The listing builds one solid part. Answer for the finished solid, in the listing's coordinates (mm). Face numbers are marked on the shaded views. A direction names the side the tool comes from. Coordinates: 2 decimals unless noted, no trailing zeros. Write each loop counter-clockwise with the first axis right and the second up, starting at its lowest first coordinate (ties: lowest second). Pieces come first, ordered by that corner, then holes. Notation, with made-up numbers: M -23,37 L 5,37 A9 ccw 5,53 Z; hole C 22.25,-36.75 d11. An arc over 180 degrees is marked long. Answer as a JSON object with one key per item and string values. Group by question number.
from build123d import *

# Parameters (mm, degrees)
F1_DEPTH = 60
F2_W     = 70
F2_H     = 15
F3_DEPTH = 50
F4_R     = 15
F5_R     = 15
F6_DEPTH = 67.5
F7_SIZE  = 5
F8_SIZE  = 4.99999
F9_SIZE  = 5


# Not quite as in the source:
# - a fillet or chamfer is up to 0.001 mm smaller than in the source, because OpenCascade refuses the exact size


with BuildPart() as f1:
    # F0 (on Front) → F1 (new body)
    with BuildSketch(Plane.XZ):
        Polygon((-8.0390890029, 59.2476050396), (-48.0390890029, 59.2476050396), (-48.0390890029, -60.7523949604), (-8.0390890029, -60.7523949604), (-8.0390890029, -20.7523949604), (11.9609109971, -20.7523949604), (11.9609109971, -60.7523949604), (51.9609109971, -60.7523949604), (51.9609109971, 59.2476050396), (11.9609109971, 59.2476050396), (11.9609109971, 19.2476050396), (-8.0390890029, 19.2476050396), align=None)
    extrude(amount=F1_DEPTH)

    # F2 (on face) → F3 (cut)
    with BuildSketch(Plane.XZ.offset(60)):
        with Locations((1.9609109971, -0.7523949604)):
            Rectangle(F2_W, F2_H)
    extrude(amount=-F3_DEPTH, mode=Mode.SUBTRACT)

    # F4 (on face) + F5 (on face) → F6 (cut)
    with BuildSketch(Plane(origin=(0, 0, -60.7523949604), x_dir=(1, 0, 0), z_dir=(0, 0, -1))):
        with Locations((-28.0390890029, 20)):
            Circle(F4_R)
    with BuildSketch(Plane(origin=(0, 0, -60.7523949604), x_dir=(1, 0, 0), z_dir=(0, 0, -1))):
        with Locations((31.9609109971, 20)):
            Circle(F5_R)
    extrude(amount=-F6_DEPTH, mode=Mode.SUBTRACT)

    # F7
    f7_edges = [f1.edges().sort_by_distance(p)[0] for p in [
        (-48.039089, -30, 59.247605),
        (-8.039089, -30, 59.247605),
        (11.960911, -30, 59.247605),
        (51.960911, -30, 59.247605),
        (31.960911, -60, 59.247605),
        (-28.039089, -60, 59.247605),
        (31.960911, 0, 59.247605),
        (-28.039089, 0, 59.247605),
        (1.960911, -60, 6.747605),
        (-33.039089, -60, -0.752395),
        (1.960911, -60, -8.252395),
        (36.960911, -60, -0.752395),
        (51.960911, -60, -0.752395),
        (51.960911, 0, -0.752395),
        (11.960911, -60, 39.247605),
        (1.960911, -60, 19.247605),
        (-8.039089, -60, 39.247605),
        (31.960911, -60, -60.752395),
        (11.960911, -60, -40.752395),
        (-48.039089, -60, -0.752395),
        (1.960911, -60, -20.752395),
        (-28.039089, -60, -60.752395),
        (-8.039089, -60, -40.752395),
        (-48.039089, 0, -0.752395),
        (11.960911, 0, -40.752395),
        (-8.039089, 0, -40.752395),
        (11.960911, 0, 39.247605),
        (-8.039089, 0, 39.247605),
    ]]
    chamfer(f7_edges, length=F7_SIZE)

    # F8 (size 5 in the source; OpenCascade refuses exactly that, so slightly less here)
    f8_edges = [f1.edges().sort_by_distance(p)[0] for p in [
        (1.960911, 0, -20.752395),
    ]]
    chamfer(f8_edges, length=F8_SIZE)

    # F9
    f9_edges = [f1.edges().sort_by_distance(p)[0] for p in [
        (1.960911, 0, 19.247605),
    ]]
    chamfer(f9_edges, length=F9_SIZE)


solid = f1.part
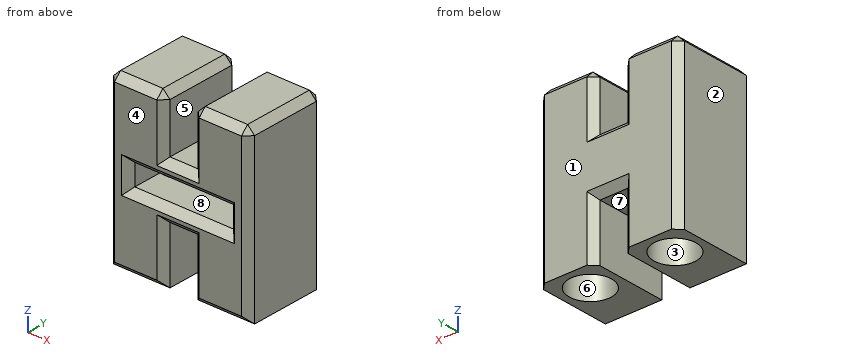
Item 1: Consider L1, parallel to X at y = -20, z = -32; L2, parallel to X at y = -20, z = -10.5; L3, parallel to X at y = -20, z = 19.5. Determine where each line is inside the solid, lowest interval first. Write a range as from..to.
Item 2: For a pull along Y with two mould halves and no side action, classify the marked faces 1, 2, 3 and 4 as +Y half, -Y half, draft (parallel to the pull), parting line (faces both ways), or undercut.
Item 3: A cutting plane is placed at C-C, the plane z = 30. Write down the section's boundary in (x, y), and give its area (3 significant figures).
Item 4: A cutting plane is placed at A-A, the plane z = -38. Write down the section's boundary in (x, y).
Item 5: A cutting plane is placed at B-B, the plane y = -20. Write down the section's boundary in (x, z).
Item 6: Flat-ended cylindrical pins translate along their axes: pin 1 Ø22 at (x, y) = (3, -40) entering from +Z; pin 2 Ø10 at (x, y) = (-3, -33.5) entering from -Z; pin 3 Ø12 at (x, z) = (-6.5, -3) entering from -Y. Find the tip coordinate at first contact, or state that the pin passes through.
Item 7: A tool of negligible diameter and unlimited length cuts with its end or side. For the marked faces 5, 6, 7 and 8, from which of +Z, -Z, +X, -X, +Y, -Y can it reach the whole face along a straight path? Write none if from no direction.
Item 8: A cutting plane is placed at D-D, the plane x = -29.5. Write down the section's boundary in (y, z).
Answer:
{
 "1": {"L1": "-48.04..-43.04, -13.04..-8.04, 11.96..16.96, 46.96..51.96", "L2": "-48.04..-43.04, -13.04..16.96, 46.96..51.96", "L3": "-48.04..-8.04, 11.96..51.96"},
 "2": {"face 1": "+Y half", "face 2": "draft", "face 3": "undercut", "face 4": "-Y half"},
 "3": {"outline": "M -48.04,-55 L -43.04,-60 L -13.04,-60 L -8.04,-55 L -8.04,-5 L -13.04,0 L -43.04,0 L -48.04,-5 Z; M 11.96,-55 L 16.96,-60 L 46.96,-60 L 51.96,-55 L 51.96,-5 L 46.96,0 L 16.96,0 L 11.96,-5 Z", "area": "4,700 mm2"},
 "4": {"outline": "M -48.04,-55 L -43.04,-60 L -13.04,-60 L -8.04,-55 L -8.04,-5 L -13.04,0 L -43.04,0 L -48.04,-5 Z; M 11.96,-55 L 16.96,-60 L 46.96,-60 L 51.96,-55 L 51.96,-5 L 46.96,0 L 16.96,0 L 11.96,-5 Z; hole C -28.04,-20 d30; hole C 31.96,-20 d30"},
 "5": {"outline": "M -48.04,-60.75 L -43.04,-60.75 L -43.04,6.75 L 46.96,6.75 L 46.96,-60.75 L 51.96,-60.75 L 51.96,54.25 L 46.96,59.25 L 16.96,59.25 L 11.96,54.25 L 11.96,19.25 L -8.04,19.25 L -8.04,54.25 L -13.04,59.25 L -43.04,59.25 L -48.04,54.25 Z; M -13.04,-60.75 L -8.04,-60.75 L -8.04,-20.75 L 11.96,-20.75 L 11.96,-60.75 L 16.96,-60.75 L 16.96,-8.25 L -13.04,-8.25 Z"},
 "6": {"pin 1": "z = 56.29", "pin 2": "z = -20.75", "pin 3": "y = -55.75"},
 "7": {"face 5": "+Z, +Y, -Y", "face 6": "-Z", "face 7": "-Z, +Y, -Y", "face 8": "-Y"},
 "8": {"outline": "M -60,-55.75 L -55,-60.75 L -34.93,-60.75 L -34.93,-8.25 L -55,-8.25 L -60,-13.25 Z; M -60,11.75 L -55,6.75 L -5.07,6.75 L -5.07,-60.75 L 0,-60.75 L 0,54.25 L -5,59.25 L -55,59.25 L -60,54.25 Z"}
}
